Could you check a few things on this model? Use its own coordinates, in mm. Face numbers are marked on the shaded views. A direction names the side the tool comes from. Round coordinates to 2 decimals unless told otherwise and drop trailing zeros. Order: outer loops, then holes, each group sorted by start corner. A loop starts at its lowest first (then second) coordinate and runs counter-clockwise, first axis right, second up. Notation, with made-up numbers: (68, 5) -> (81, 5) arc R36 cw to (81, 42) -> close; hole circle Ø8 at (30.25, 31.25). An arc over 180 degrees is marked (long way). Put each result on its own line as item: value. Start each with the question number.
from build123d import *

# Parameters (mm, degrees)
MOVE_FACE2_BY                   = 0.025
DOME1_FACE_RADIUS               = 2.975
DOME1_HEIGHT                    = 0.5
FILLET1_R                       = 0.5
SKETCH2_R                       = 0.75
BOSS_EXTRUDE1_DEPTH             = 3.45
SKETCH3_W                       = 4
SKETCH3_H                       = 1
EXTRUDE_THIN1_DEPTH             = 3.45
MOVE_FACE1_BY                   = 0.05
BOSS_EXTRUDE2_REACH             = 8.95
SKETCH4_R                       = 2
BOSS_EXTRUDE2_DIRECTION_2_REACH = 8.95


with BuildPart() as part:
    # Sketch1 → Revolve1 (revolve)
    with BuildSketch(Plane(origin=(0, 0, 0), x_dir=(0, 0, -1), z_dir=(1, 0, 0))):
        Polygon((0, 2.236067977), (3, 2.236067977), (3, -1.039151263), (3.5, -1.039151263), (3.5, -2.539151263), (2, -2.539151263), (2, 1.236067977), (0, 1.236067977), align=None)
    revolve(axis=Axis((0, 1.236067977, 0), (0, 1, 0)))

    # Move Face2: a curved face moved inward by 0.025
    add(Solid.thicken(part.faces().sort_by_distance((0, 0.598458357, 3))[0], -MOVE_FACE2_BY), mode=Mode.SUBTRACT)

    # Dome1: a dome of height H over a round flat face of radius A is a cap of a sphere of radius (A * A + H * H) / (2 * H)
    dome1_r = (DOME1_FACE_RADIUS * DOME1_FACE_RADIUS + DOME1_HEIGHT * DOME1_HEIGHT) / (2 * DOME1_HEIGHT)
    dome1_base = Plane((0, 2.236067977, 0), z_dir=(0, 1, 0))
    with Locations(dome1_base.offset(DOME1_HEIGHT - dome1_r)):
        dome1_ball = Sphere(dome1_r, mode=Mode.PRIVATE)
    add(split(dome1_ball, bisect_by=dome1_base, keep=Keep.TOP, mode=Mode.PRIVATE))

    # Fillet1
    fillet1_edges = [part.edges().sort_by_distance(p)[0] for p in [
        (2.975, 2.236067977, 0),
    ]]
    fillet(fillet1_edges, radius=FILLET1_R)

    # Sketch2 → Boss-Extrude1 (add)
    with BuildSketch(Plane.XZ.offset(-1.236067977)):
        with Locations(Location((0, 0, 0), (0, 0, 90))):
            Circle(SKETCH2_R)
    extrude(amount=BOSS_EXTRUDE1_DEPTH)

    # Sketch3 → Extrude-Thin1 (add)
    with BuildSketch(Plane.XZ.offset(2.213932023)):
        Rectangle(SKETCH3_W, SKETCH3_H)
    extrude(amount=-EXTRUDE_THIN1_DEPTH)

    # Move Face1: a curved face moved inward by 0.05
    add(Solid.thicken(part.faces().sort_by_distance((0, -1.789151263, 3.5))[0], -MOVE_FACE1_BY), mode=Mode.SUBTRACT)

    # Sketch4 → Boss-Extrude2 (add, up to next)
    with BuildSketch(Plane.XZ.offset(2.213932023), mode=Mode.PRIVATE) as boss_extrude2_sk1:
        Circle(SKETCH4_R)
    boss_extrude2_tool1 = extrude(boss_extrude2_sk1.sketch, amount=-BOSS_EXTRUDE2_REACH, mode=Mode.PRIVATE) - part.part
    add(boss_extrude2_tool1.solids().sort_by_distance((0, -2.213932, 0))[0])
    add(boss_extrude2_tool1.solids().sort_by_distance((0, -2.213932, 0))[1])

    # Boss-Extrude2 direction 2: up to this face of the body (flat: up to its plane)
    boss_extrude2_direction_2_end = Plane(part.part.faces().sort_by_distance((0, -2.539151263, 3.352419264))[0])
    # Sketch4 → Boss-Extrude2 direction 2 (add, up to the picked face)
    with BuildSketch(Plane.XZ.offset(2.213932023), mode=Mode.PRIVATE) as boss_extrude2_direction_2_sk1:
        Circle(SKETCH4_R)
    boss_extrude2_direction_2_tool1 = split(extrude(boss_extrude2_direction_2_sk1.sketch, amount=BOSS_EXTRUDE2_DIRECTION_2_REACH, mode=Mode.PRIVATE), bisect_by=boss_extrude2_direction_2_end, keep=Keep.BOTH, mode=Mode.PRIVATE)
    add(boss_extrude2_direction_2_tool1.solids().sort_by(Axis((0, -2.213932, 0), (0, -1, 0)))[0])


solid = part.part
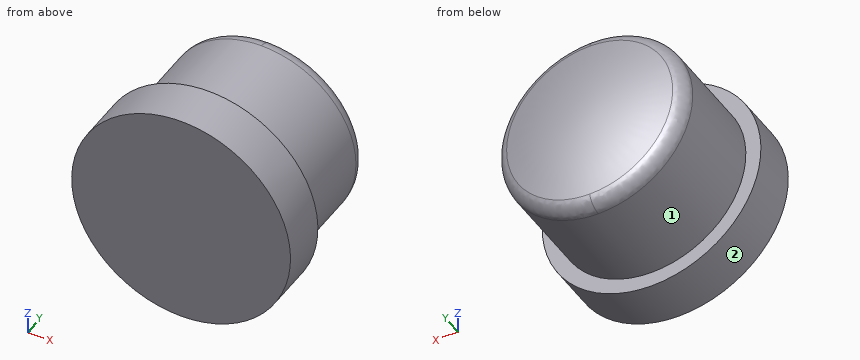
1. Which directions (+Z, -Z, +X, -X, +Y, -Y) give clear straight access to the entire face, cutting with the end or side of a thin tool? Please do the marked faces 1 and 2.
2. I need wall thicknesses on L1, parallel to Y at x = 2.25, z = 2; L2, parallel to Z at x = 1.75, y = -2.25; L3, parallel to X at y = -1.55, z = 2. Which ranges of each line are inside material? Lowest first, please.
3. If we section it at A-A, the plane y = -1.8: Please give me the cut outline in (x, z), then the cut area to 3 significant figures.
4. If we section it at B-B, the plane y = 1.75: Please give me the cut outline in (x, z) (3 decimals).
5. For pin 1 Ø1.5 at (x, z) = (-2.5, -0.5) entering from +Y; pin 2 Ø2 at (x, z) = (-1.5, -1.5) entering from +Y; pin 3 Ø2 at (x, y) = (2, -1) entering from +Z; pin 4 Ø3 at (x, y) = (1.5, -2) entering from +Z, each with a flat end and sliding along its axis, tell me the tip position at first contact or that it passes through.
Results below:
1. face 1: +Y
1. face 2: +Y, -Y
2. L1: -2.54 to -1.04
2. L2: -2.97 to 2.97
2. L3: -2.81 to 2.81
3. outline: circle Ø6.9 at (0, 0)
3. area: 37.4 mm2
4. outline: circle Ø5.95 at (0, 0)
5. pin 1: y = 2.56
5. pin 2: y = 2.67
5. pin 3: z = 3.3
5. pin 4: z = 3.45
